Part model, mm, in its own coordinate system. A direction names the side the tool comes from. Round coordinates to 2 decimals unless told otherwise and drop trailing zeros. Write each loop counter-clockwise with the first axis right and the second up, starting at its lowest first coordinate (ties: lowest second). Pieces come first, ordered by that corner, then holes. Notation, with made-up numbers: (4.5, 38) -> (40.5, 38) arc R28 cw to (40.5, 72) -> close; hole circle Ø3 at (-15, -4.5). An arc over 180 degrees is marked (long way). Use CSV: the item, a comma, the result in double quotes. Start each with the question number.
(1) Saw through at D-D (y = 39.5). Give the cut face in (x, z).
(2) Two-plate mould, pull along X, no slides. Class faces 1 (the flat face through (1, 93, 6.35)), 2 (the cylindrical face through (123.98, 54.79, 3.22)), 3 (the cylindrical face through (-130.193, 37.725, 3.219)), 4 (the cylindrical face through (0.103, 99.776, 3.131)): released by +X, released by -X, zero draft, split by the parting line, or undercut.
(3) Saw through at C-C (y = 85). Give the cut face in (x, z).
(4) Drop flat-ended pins along their axis: pin 1 (1.5 mm diameter, centred on x = 59, z = 2.5, fed in from -Y); pin 2 (1 mm diameter, centred on x = -77.5, z = 1, fed in from -Y); pin 3 (3 mm diameter, centred on y = 108, z = 4, fed in from +X). Give the stop position or say it passes through.
(5) Probe line 1 (X direction, y = 105, z = 2.25); line 2 (Y direction, x = -3.5, z = 1); line 3 (X direction, y = 46, z = 0.5). List the from-to ranges inside material, lowest first. Write a range as [from, to].
(6) Saw through at A-A (y = 114). Give the cut face in (x, z).
(7) Which spindle directions (+Z, -Z, +X, -X, +Y, -Y) get a long thin tool onto all of the face, cutting with end or side? Do faces 5 (the flat face through (4.762, 111, 3)), 6 (the flat face through (1, 93, 0)), 7 (the cylindrical face through (-84.476, 67.209, 3.131)). Say none if no direction does.
```python
from build123d import *

# Parameters (mm, degrees)
BOSS_EXTRUDE1_DEPTH     = 6.35
FILLET1_R               = 12.7
CUT_EXTRUDE1_DEPTH      = 192.457982885
CUT_EXTRUDE1_DEPTH_BACK = 192.457982885


with BuildPart() as part:
    # Sketch1 → Boss-Extrude1 (new body)
    with BuildSketch(Plane.XY):
        with BuildLine():
            Line((-12.7, 126.363404513), (-12.7, 139.063404513))
            Line((-12.7, 139.063404513), (12.7, 139.063404513))
            Line((12.7, 139.063404513), (12.7, 126.363404513))
            ThreePointArc((12.7, 126.363404513), (72.844207417, 104.032309625), (114.399102938, 55.152926006))
            Line((114.399102938, 55.152926006), (126.333199222, 59.496581827))
            Line((126.333199222, 59.496581827), (135.020510862, 35.628389259))
            Line((135.020510862, 35.628389259), (123.086414578, 31.284733439))
            ThreePointArc((123.086414578, 31.284733439), (123.187942798, 30.882531456), (123.288156771, 30.48))
            Line((123.288156771, 30.48), (103.55757867, 30.48))
            ThreePointArc((103.55757867, 30.48), (84.832852027, 66.757694065), (53.975, 93.487442339))
            Line((53.975, 93.487442339), (44.45, 76.989658396))
            ThreePointArc((44.45, 76.989658396), (0, 88.9), (-44.45, 76.989658396))
            Line((-44.45, 76.989658396), (-53.975, 93.487442339))
            ThreePointArc((-53.975, 93.487442339), (-84.832852027, 66.757694065), (-103.55757867, 30.48))
            Line((-103.55757867, 30.48), (-123.288156771, 30.48))
            ThreePointArc((-123.288156771, 30.48), (-123.187942798, 30.882531456), (-123.086414578, 31.284733439))
            Line((-123.086414578, 31.284733439), (-135.020510862, 35.628389259))
            Line((-135.020510862, 35.628389259), (-126.333199222, 59.496581827))
            Line((-126.333199222, 59.496581827), (-114.399102938, 55.152926006))
            ThreePointArc((-114.399102938, 55.152926006), (-72.844207417, 104.032309625), (-12.7, 126.363404513))
        make_face()
    extrude(amount=BOSS_EXTRUDE1_DEPTH)

    # Fillet1
    fillet1_edges = [part.edges().sort_by_distance(p)[0] for p in [
        (135.020510862, 35.628389259, 3.175),
        (126.333199222, 59.496581827, 3.175),
        (-135.020510862, 35.628389259, 3.175),
        (-126.333199222, 59.496581827, 3.175),
        (-12.7, 139.063404513, 3.175),
        (12.7, 139.063404513, 3.175),
    ]]
    fillet(fillet1_edges, radius=FILLET1_R - 0.0001)  # a hair under: the kernel refuses the full size

    # Sketch2 → Cut-Extrude1 (cut, two sides: drawn at the far end of the back side and taken through both)
    with BuildSketch(Plane.XY.offset(6.35).offset(-CUT_EXTRUDE1_DEPTH_BACK)):
        with BuildLine():
            Line((-4.762498, 104.541870481), (-4.762498, 117.241865148))
            ThreePointArc((-4.762498, 117.241865148), (0.002182277, 122.000000094), (4.7625, 117.237500594))
            Line((4.7625, 117.237500594), (4.7625, 104.537500594))
            ThreePointArc((4.7625, 104.537500594), (-0.002184944, 99.77500109), (-4.762498, 104.541870481))
        make_face()
    extrude(amount=CUT_EXTRUDE1_DEPTH + CUT_EXTRUDE1_DEPTH_BACK, mode=Mode.SUBTRACT)


solid = part.part
```
Answers:
1,outline,"(-130.89, 0) -> (-100.46, 0) -> (-100.46, 6.35) -> (-130.89, 6.35) -> close; (100.46, 0) -> (130.89, 0) -> (130.89, 6.35) -> (100.46, 6.35) -> close"
2,face 1,"zero draft"
2,face 2,"undercut"
2,face 3,"released by -X"
2,face 4,"undercut"
3,outline,"(-94.36, 0) -> (-66.54, 0) -> (-66.54, 6.35) -> (-94.36, 6.35) -> close; (-49.07, 0) -> (-26.04, 0) -> (-26.04, 6.35) -> (-49.07, 6.35) -> close; (26.04, 0) -> (49.07, 0) -> (49.07, 6.35) -> (26.04, 6.35) -> close; (66.54, 0) -> (94.36, 0) -> (94.36, 6.35) -> (66.54, 6.35) -> close"
4,pin 1,"stops at y = 89.91"
4,pin 2,"stops at y = 74.63"
4,pin 3,"stops at x = 69.19"
5,line 1,"x = [-71.44, -4.76], [4.76, 71.44]"
5,line 2,"y = [88.83, 101.31], [120.47, 138.57]"
5,line 3,"x = [-131.13, -97.66], [97.66, 131.13]"
6,outline,"(-55.97, 0) -> (-4.76, 0) -> (-4.76, 6.35) -> (-55.97, 6.35) -> close; (4.76, 0) -> (55.97, 0) -> (55.97, 6.35) -> (4.76, 6.35) -> close"
7,face 5,"+Z, -Z"
7,face 6,"-Z, +X, -X, +Y, -Y"
7,face 7,"+Z, -Z, -Y"
